Geometry: see drawing. Coordinates: mm, zero at the bounding-box minimum. A direction names the side the tool comes from. Coordinates: 2 decimals unless noted, no trailing zeros. Write each loop counter-clockwise with the first axis right and the second up, starting at its lowest first coordinate (ties: lowest second). Pieces come first, ordered by that corner, then holes. Notation, with made-up numbers: M 53,69.5 L 62,69.5 A24 cw 62,83.5 Z; hole C 72,-19 d9. An arc over 180 degrees is marked long. Answer as CSV lines item,"result". Start each with the question number.
1. Contact query for flat-ended pins moving along their axis: pin 1 Ø0.9 at (y, z) = (10, 59.5) entering from +X; pin 2 Ø1.5 at (x, z) = (56, 34) entering from -Y (3 decimals); pin 3 Ø2 at (y, z) = (13.5, 61) entering from +X. Output: stop coordinate, or through.
2. Section D-D on x = 10.16. Return the cut outline in (y, z) (3 decimals), plus the area to 3 significant figures.
3. Section B-B on z = 34. Return the cut outline in (x, y) (3 decimals), plus the area to 3 significant figures.
4. Section A-A on x = 48. Return the cut outline in (y, z) (3 decimals).
5. Mould query, pull axis Z, two halves, no side actions, for the marked faces 3, 4 and 5. Classes: pulls with the +Z half, pulls with the -Z half, needs draft (parallel to the pull), parting line crosses it, or undercut.
6. Line query: probe 1 along Z at (x, y) = (66, 3); probe 2 along Y at (x, z) = (34, 16.5) (3 decimals); probe 3 along Z at (x, y) = (36.5, 15). Output: solid intervals per line, ascending. Write a range as [from, to].
7. Section C-C on z = 3.81. Return the cut outline in (x, y) (3 decimals).
8. Reachability of the marked faces 1 and 2 from +Z, -Z, +X, -X, +Y, -Y: full face, straight path, thin tool, end or side. Return the list, or none.
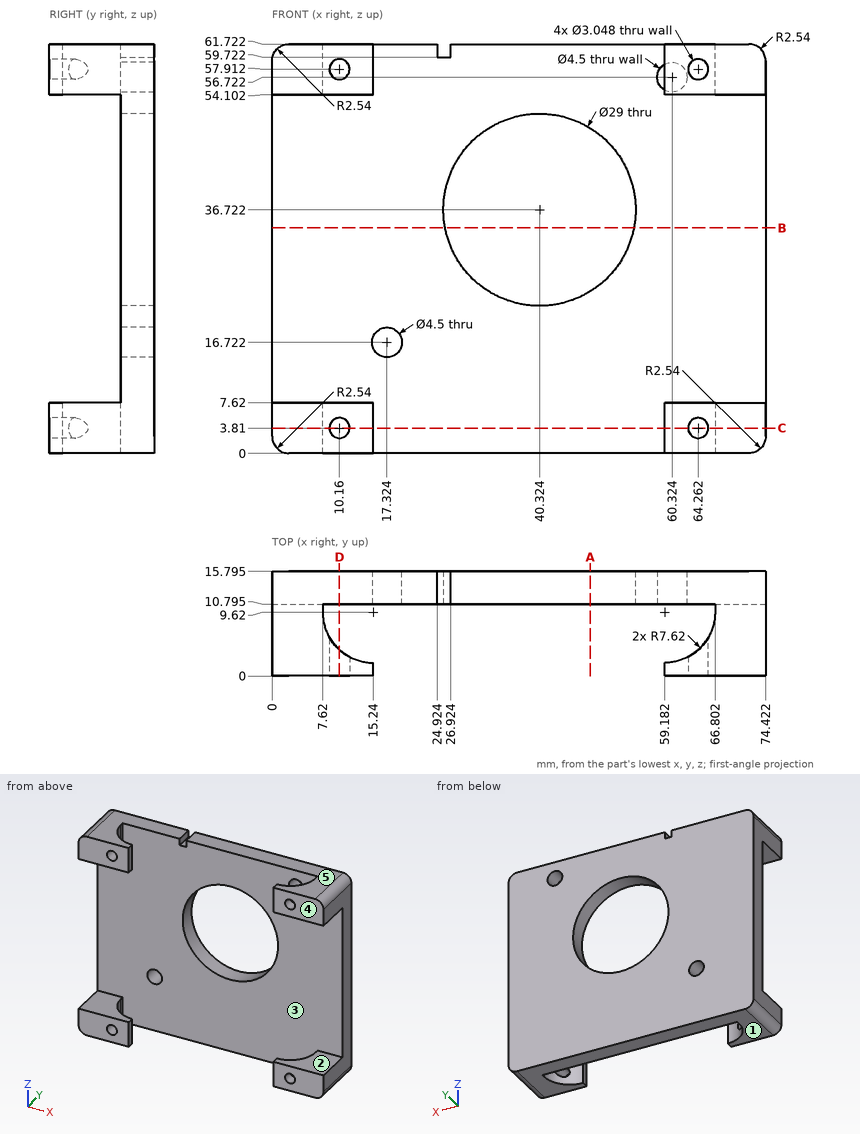
Values:
1,pin 1,"x = 74.42"
1,pin 2,"y = 10.795"
1,pin 3,"x = 74.29"
2,outline,"M 0,0 L 3.94,0 L 3.94,2.286 L 0,2.286 Z; M 0,5.334 L 3.94,5.334 L 3.94,7.62 L 0,7.62 Z; M 0,54.102 L 3.94,54.102 L 3.94,56.388 L 0,56.388 Z; M 0,59.436 L 3.94,59.436 L 3.94,61.722 L 0,61.722 Z; M 10.795,0 L 15.795,0 L 15.795,61.722 L 10.795,61.722 Z"
2,area,"345 mm²"
3,outline,"M 0,10.795 L 26.082,10.795 L 26.082,15.795 L 0,15.795 Z; M 54.566,10.795 L 74.422,10.795 L 74.422,15.795 L 54.566,15.795 Z"
3,area,"230 mm²"
4,outline,"M 10.795,0 L 15.795,0 L 15.795,24.42 L 10.795,24.42 Z; M 10.795,49.024 L 15.795,49.024 L 15.795,61.722 L 10.795,61.722 Z"
5,face 3,"undercut"
5,face 4,"needs draft"
5,face 5,"pulls with the +Z half"
6,probe 1,"[0, 7.62], [54.1, 61.72]"
6,probe 2,"[10.795, 15.795]"
6,probe 3,"[0, 22.74], [50.71, 61.72]"
7,outline,"M 0,0 L 8.636,0 L 8.636,5.818 A7.62 cw 7.62,9.62 L 7.62,10.795 L 66.802,10.795 L 66.802,9.62 A7.62 cw 65.786,5.818 L 65.786,0 L 74.422,0 L 74.422,15.795 L 0,15.795 Z; M 11.684,0 L 15.24,0 L 15.24,2 A7.62 cw 11.684,2.881 Z; M 59.182,0 L 62.738,0 L 62.738,2.881 A7.62 cw 59.182,2 Z"
8,face 1,"-Z, +X, -X, +Y, -Y"
8,face 2,"+X, -X, -Y"
